```python
from build123d import *

# Parameters (mm, degrees)
SKETCH1_W           = 228.6
SKETCH1_H           = 19.05
BOSS_EXTRUDE1_DEPTH = 4.7625
SKETCH2_R           = 3.175
CUT_EXTRUDE1_DEPTH  = 5.7625
SKETCH3_R           = 6.858
CUT_EXTRUDE2_DEPTH  = 5.7625
SKETCH4_R           = 3.175
CUT_EXTRUDE3_DEPTH  = 5.7625


with BuildPart() as part:
    # Sketch1 → Boss-Extrude1 (new body)
    with BuildSketch(Plane(origin=(0, 0, 0), x_dir=(1, 0, 0), z_dir=(0, 1, 0))):
        Rectangle(SKETCH1_W, SKETCH1_H)
    extrude(amount=BOSS_EXTRUDE1_DEPTH)

    # Sketch2 → Cut-Extrude1 (cut, through all)
    with BuildSketch(Plane(origin=(0, 4.7625, 0), x_dir=(1, 0, 0), z_dir=(0, 1, 0))):
        with Locations(Location((102.39375, 0, 0), (0, 0, 270))):  # turned: the seam where the file's is
            Circle(SKETCH2_R)
        with Locations(Location((-102.39375, 0, 0), (0, 0, 90))):  # turned: the seam where the file's is
            Circle(SKETCH2_R)
    extrude(amount=-CUT_EXTRUDE1_DEPTH, mode=Mode.SUBTRACT)

    # Sketch3 → Cut-Extrude2 (cut, through all)
    with BuildSketch(Plane(origin=(0, 4.7625, 0), x_dir=(1, 0, 0), z_dir=(0, 1, 0))):
        with Locations((-86.614, 9.525)):
            Circle(SKETCH3_R)
    extrude(amount=-CUT_EXTRUDE2_DEPTH, mode=Mode.SUBTRACT)

    # Sketch4 → Cut-Extrude3 (cut, through all)
    with BuildSketch(Plane(origin=(0, 4.7625, 0), x_dir=(1, 0, 0), z_dir=(0, 1, 0))):
        with Locations(Location((-66.3575, 0, 0), (0, 0, 270))):  # turned: the seam where the file's is
            Circle(SKETCH4_R)
        with Locations(Location((66.3575, 0, 0), (0, 0, 270))):  # turned: the seam where the file's is
            Circle(SKETCH4_R)
    extrude(amount=-CUT_EXTRUDE3_DEPTH, mode=Mode.SUBTRACT)


solid = part.part
```
Build history of the part. All positions in model axes, mm. Give positions to 0.01 mm unless a question says otherwise; leave off trailing zeros. Loops run counter-clockwise (first coordinate to the right, second up) from the corner with the lowest first, then second, coordinate; pieces in that order, holes last. Notation, with made-up numbers: (6.25, 81.5) -> (51.25, 81.5) arc R25 cw to (51.25, 116.5) -> close; hole circle Ø3 at (79.25, 84.5). An arc over 180 degrees is marked (long way). One line per question, with ' | ' between items. Start each with the question number.
1) Pin check, flat tip, straight feed: pin 1 (5 mm diameter, centred on x = 66.36, z = 0, fed in from -Y). Stop position of the tip, or through.
2) Two-plate mould, pull along X, no slides. Class faces 1 (the cylindrical face through (-63.68, 2.41, 1.71)), 2 (the flat face through (-114.3, 2, 0)), 3 (the flat face through (-2, 0, 0)): released by +X, released by -X, zero draft, split by the parting line, or undercut.
3) Probe L1, parallel to X at y = 1.1, z = 0; L2, parallel to X at y = 1.9, z = -0.5; L3, parallel to Z at x = -84, y = 3.35 (3 decimals). List the from-to ranges inside material, lowest first.
4) Cut at A-A (z = 0). Give the cut face in (x, y), plus the area to 3 significant figures.
5) Cut at B-B (y = 1.15). Count the separate pieces of the cut face and the enclosed holes in it, plus the area to 3 significant figures.
Return value:
1) pin 1: through
2) face 1: undercut | face 2: released by -X | face 3: zero draft
3) L1: -114.3 to -105.57, -99.22 to -69.53, -63.18 to 63.18, 69.53 to 99.22, 105.57 to 114.3 | L2: -114.3 to -105.53, -99.26 to -69.49, -63.22 to 63.22, 69.49 to 99.26, 105.53 to 114.3 | L3: -3.185 to 9.525
4) outline: (-114.3, 0) -> (-105.57, 0) -> (-105.57, 4.76) -> (-114.3, 4.76) -> close; (-99.22, 0) -> (-69.53, 0) -> (-69.53, 4.76) -> (-99.22, 4.76) -> close; (-63.18, 0) -> (63.18, 0) -> (63.18, 4.76) -> (-63.18, 4.76) -> close; (69.53, 0) -> (99.22, 0) -> (99.22, 4.76) -> (69.53, 4.76) -> close; (105.57, 0) -> (114.3, 0) -> (114.3, 4.76) -> (105.57, 4.76) -> close | area: 968 mm^2
5) separate pieces: 1 | enclosed holes: 4 | area: 4,150 mm^2
